from build123d import *

# Parameters (mm, degrees)
SKETCH1_W            = 62.28
SKETCH1_H            = 2.98
BOSS_EXTRUDE1_DEPTH  = 155.03
SKETCH2_W            = 7.5
SKETCH2_H            = 40
CUT_EXTRUDE1_DEPTH   = 159.154610745
FILLET1_R            = 1
FILLET1_OF_MIRROR1_R = 1


with BuildPart() as part:
    # Sketch1 → Boss-Extrude1 (new body)
    with BuildSketch(Plane(origin=(0, 0, 0), x_dir=(0, 0, -1), z_dir=(1, 0, 0))):
        Rectangle(SKETCH1_W, SKETCH1_H)
    extrude(amount=BOSS_EXTRUDE1_DEPTH)

    # Sketch2 → Cut-Extrude1 (cut, through all)
    with BuildSketch(Plane(origin=(0, 1.49, 0), x_dir=(1, 0, 0), z_dir=(0, 1, 0))):
        with Locations((9.795259857, -11.14)):
            Rectangle(SKETCH2_W, SKETCH2_H)
    cut_extrude1 = extrude(amount=-CUT_EXTRUDE1_DEPTH, mode=Mode.SUBTRACT)

    # Fillet1
    fillet1_edges = [part.edges().sort_by_distance(p)[0] for p in [
        (13.545259857, -1.49, 11.14),
        (6.045259857, -1.49, 11.14),
        (9.795259857, -1.49, -8.86),
        (13.545259857, 1.49, 11.14),
        (9.795259857, 1.49, -8.86),
        (6.045259857, 1.49, 11.14),
    ]]
    fillet(fillet1_edges, radius=FILLET1_R)

    # Mirror1: Cut-Extrude1 across plane
    add(cut_extrude1.mirror(Plane(origin=(77.515, 0, 0), x_dir=(0, 0, 1), z_dir=(1, 0, 0))), mode=Mode.SUBTRACT)

    # Fillet1 of Mirror1
    fillet1_of_mirror1_edges = [part.edges().sort_by_distance(p)[0] for p in [
        (141.484740143, -1.49, 11.14),
        (148.984740143, -1.49, 11.14),
        (145.234740143, -1.49, -8.86),
        (141.484740143, 1.49, 11.14),
        (145.234740143, 1.49, -8.86),
        (148.984740143, 1.49, 11.14),
    ]]
    fillet(fillet1_of_mirror1_edges, radius=FILLET1_OF_MIRROR1_R)


solid = part.part
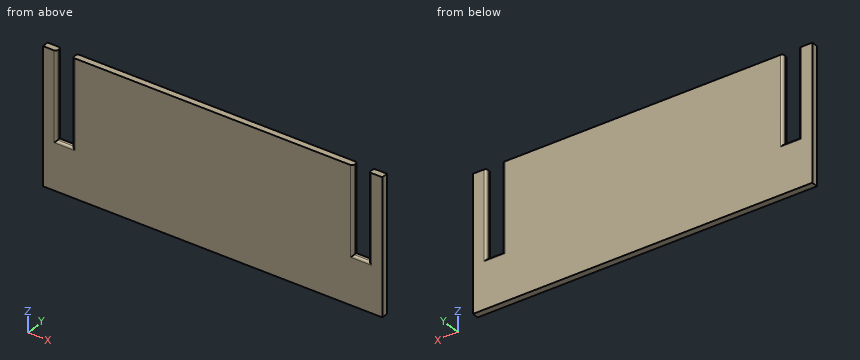
The listing builds one solid part. Answer for the finished solid, in the listing's coordinates (mm). Round coordinates to 2 decimals unless told otherwise and drop trailing zeros. Order: outer loops, then holes, each group sorted by start corner. A loop starts at its lowest first (then second) coordinate and runs counter-clockwise, first axis right, second up. Notation, with made-up numbers: M -17,33 L -6,33 A22 ccw -6,56 Z; hole C 4,-25 d8. An arc over 180 degrees is marked long. Answer in a Markdown table with one row per item. Add a question column.
1) Consider line 1 along X through (y, z) = (0.5, 12); line 2 along X through (y, z) = (-0.7, 6); line 3 along Z through (x, y) = (144, -0.2). Determine where each line is inside the solid, lowest interval first. Write a range as from..to.
2) Flat-ended cylindrical pins translate along their axes: pin 1 Ø1.1 at (y, z) = (0, 7) entering from -X; pin 2 Ø0.5 at (x, y) = (11.5, 0) entering from +Z. Find the tip coordinate at first contact, or state that the pin passes through.
3) The part is cut by section A-A on z = 18. Determine the outline of the cut face in (x, y), plus the area to 3 significant figures.
Findings below:
| question | item | result |
|---|---|---|
| 1 | line 1 | x = 0..6.05, 13.55..141.48, 148.98..155.03 |
| 1 | line 2 | x = 0..6.02, 13.57..141.46, 149.01..155.03 |
| 1 | line 3 | z = -31.14..-8.86 |
| 2 | pin 1 | stops at x = 0 |
| 2 | pin 2 | stops at z = -8.86 |
| 3 | outline | M 0,-1.49 L 5.05,-1.49 A1 ccw 6.05,-0.49 L 6.05,0.49 A1 ccw 5.05,1.49 L 0,1.49 Z; M 13.55,-0.49 A1 ccw 14.55,-1.49 L 140.48,-1.49 A1 ccw 141.48,-0.49 L 141.48,0.49 A1 ccw 140.48,1.49 L 14.55,1.49 A1 ccw 13.55,0.49 Z; M 148.98,-0.49 A1 ccw 149.98,-1.49 L 155.03,-1.49 L 155.03,1.49 L 149.98,1.49 A1 ccw 148.98,0.49 Z |
| 3 | area | 416 mm² |
